Build history of the part. All positions in model axes, mm. Face numbers are marked on the shaded views. A direction names the side the tool comes from. Give positions to 0.01 mm unless a question says otherwise; leave off trailing zeros. Loops run counter-clockwise (first coordinate to the right, second up) from the corner with the lowest first, then second, coordinate; pieces in that order, holes last. Notation, with made-up numbers: M -5,49 L 11,49 A25 cw 11,72 Z; hole C 77.5,45.5 d5. An arc over 180 degrees is marked long. Answer in a Markdown table with one row per item. Add a question column.
```python
from build123d import *

# Parameters (mm, degrees)
CROQUIS1_R              = 15.25
SALIENTE_EXTRUIR2_DEPTH = 70
CROQUIS3_W              = 57
CROQUIS3_H              = 229.06918818
CORTAR_EXTRUIR1_DEPTH   = 267.557713194
CROQUIS5_R              = 10.7
SALIENTE_EXTRUIR3_DEPTH = 15
CROQUIS1_2_R            = 15.25
CORTAR_EXTRUIR2_DEPTH   = 2.5
CROQUIS7_R              = 15.25
CORTAR_EXTRUIR3_DEPTH   = 2.5


with BuildPart() as part:
    # Croquis1 → Saliente-Extruir2 (new body)
    with BuildSketch(Plane(origin=(0, 0, 0), x_dir=(0, 0, -1), z_dir=(1, 0, 0))):
        with BuildLine():
            Line((50.000039636, 19.999952763), (205.563531497, 175.563444624))
            Line((205.563531497, 175.563444624), (208.567950725, 178.567863852))
            ThreePointArc((208.567950725, 178.567863852), (211.324847557, 210.079338837), (179.813372572, 212.836235669))
            Line((179.813372572, 212.836235669), (-49.999960364, 19.999952763))
            Line((-49.999960364, 19.999952763), (-49.999960364, -20.000047237))
            Line((-49.999960364, -20.000047237), (50.000039636, -20.000047237))
            Line((50.000039636, -20.000047237), (50.000039636, 19.999952763))
        make_face()
        with Locations((194.190661648, 195.702049761)):
            Circle(CROQUIS1_R, mode=Mode.SUBTRACT)
    extrude(amount=SALIENTE_EXTRUIR2_DEPTH)

    # Croquis3 → Cortar-Extruir1 (cut, through all)
    with BuildSketch(Plane.XY.offset(49.999960364)):
        with Locations((35, 103.534546853)):
            Rectangle(CROQUIS3_W, CROQUIS3_H)
    extrude(amount=-CORTAR_EXTRUIR1_DEPTH, mode=Mode.SUBTRACT)

    # Croquis5 → Saliente-Extruir3 (add)
    with BuildSketch(Plane.XZ.offset(20.000047237)):
        with Locations((35, -3.9636e-05)):
            Circle(CROQUIS5_R)
    extrude(amount=SALIENTE_EXTRUIR3_DEPTH)

    # Croquis1_2 → Cortar-Extruir2 (cut)
    with BuildSketch(Plane(origin=(0, 0, 0), x_dir=(0, 0, -1), z_dir=(1, 0, 0))):
        with BuildLine():
            Line((50.000039636, 19.999952763), (205.563531497, 175.563444624))
            Line((205.563531497, 175.563444624), (208.567950725, 178.567863852))
            ThreePointArc((208.567950725, 178.567863852), (211.324847557, 210.079338837), (179.813372572, 212.836235669))
            Line((179.813372572, 212.836235669), (-49.999960364, 19.999952763))
            Line((-49.999960364, 19.999952763), (-49.999960364, -20.000047237))
            Line((-49.999960364, -20.000047237), (50.000039636, -20.000047237))
            Line((50.000039636, -20.000047237), (50.000039636, 19.999952763))
        make_face()
        with Locations((194.190661648, 195.702049761)):
            Circle(CROQUIS1_2_R, mode=Mode.SUBTRACT)
    extrude(amount=CORTAR_EXTRUIR2_DEPTH, mode=Mode.SUBTRACT)

    # Croquis7 → Cortar-Extruir3 (cut)
    with BuildSketch(Plane(origin=(70, 0, 0), x_dir=(0, 0, -1), z_dir=(1, 0, 0))):
        with BuildLine():
            Line((179.813372572, 212.836235669), (-49.999960364, 19.999952763))
            Line((-49.999960364, 19.999952763), (-49.999960364, -20.000047237))
            Line((-49.999960364, -20.000047237), (50.000039636, -20.000047237))
            Line((50.000039636, -20.000047237), (50.000039636, 19.999952763))
            Line((50.000039636, 19.999952763), (208.567950725, 178.567863852))
            ThreePointArc((208.567950725, 178.567863852), (211.324847557, 210.079338837), (179.813372572, 212.836235669))
        make_face()
        with Locations((194.190661648, 195.702049761)):
            Circle(CROQUIS7_R, mode=Mode.SUBTRACT)
    extrude(amount=-CORTAR_EXTRUIR3_DEPTH, mode=Mode.SUBTRACT)


solid = part.part
```
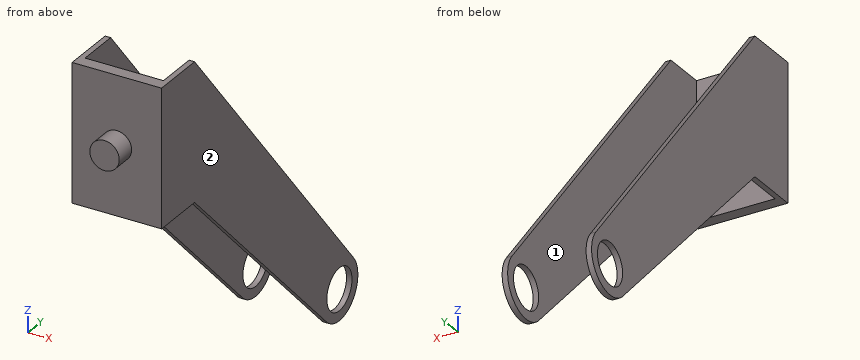
(1) Wall check: line 1 (X direction, y = 158, z = -129); line 2 (Y direction, x = 14.5, z = -24.5); line 3 (Z direction, x = 52.5, y = -15.5). Give the ranges that are in metal, low to high.
(2) Slice it at C-C, the plane z = -103. Give the cut face in (x, y).
(3) Slice it at A-A, the plane y = -1. Give the cut face in (x, z), then the cut area to 3 significant figures.
(4) Tool access for the marked faces 1 and 2: list every direction of +Z, -Z, +X, -X, +Y, -Y with a clear straight run to the whole face (end or side of a thin tool).
(5) Pin check, flat tips, straight feed: pin 1 (2 mm diameter, centred on x = 39.5, z = -46.5, fed in from -Y); pin 2 (10 mm diameter, centred on x = 10.5, z = -8.5, fed in from +Y). Stop position of each tip, or through.
(6) Slice it at B-B, the plane x = 35. Give the cut face in (y, z).
(7) Slice it at D-D, the plane z = -32.5. Give the cut face in (x, y).
Solution:
| question | item | result |
|---|---|---|
| 1 | line 1 | 2.5 to 6.5, 63.5 to 67.5 |
| 1 | line 2 | -20 to -11 |
| 1 | line 3 | -50 to 50 |
| 2 | outline | M 2.5,73 L 6.5,73 L 6.5,148.38 L 2.5,148.38 Z; M 63.5,73 L 67.5,73 L 67.5,148.38 L 63.5,148.38 Z |
| 3 | outline | M 2.5,-50 L 6.5,-50 L 6.5,50 L 2.5,50 Z; M 63.5,-50 L 67.5,-50 L 67.5,50 L 63.5,50 Z |
| 3 | area | 800 mm^2 |
| 4 | face 1 | +Z, -Z, +Y |
| 4 | face 2 | +Z, -Z, +X, +Y, -Y |
| 5 | pin 1 | y = -20 |
| 5 | pin 2 | y = 71.6 |
| 6 | outline | M -35,-10.7 L -20,-10.7 L -20,-50 L -11,-50 L -11,50 L -20,50 L -20,10.7 L -35,10.7 Z |
| 7 | outline | M 2.5,-20 L 67.5,-20 L 67.5,89.23 L 63.5,89.23 L 63.5,-11 L 6.5,-11 L 6.5,89.23 L 2.5,89.23 Z |
